Input: dimensioned drawing with shaded views. Units: mm. Origin: part minimum x, y, z. Give positions to 0.01 mm unless a question says otherwise; leave off trailing zeros. Loops run counter-clockwise (first coordinate to the right, second up) from the corner with the lowest first, then second, coordinate; pieces in that order, holes last.
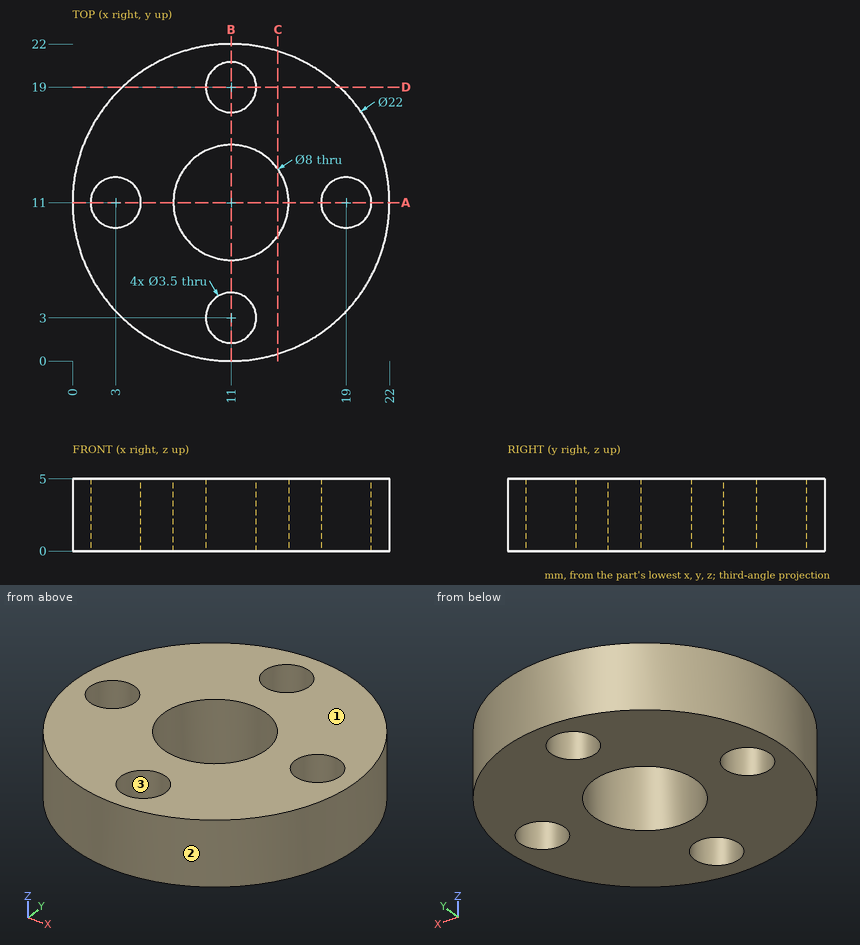
Item 1: Pin query (flat end, axial travel): pin 1 (2 mm diameter, centred on x = 6.5, z = 4, fed in from -Y); pin 2 (3 mm diameter, centred on x = 5.5, z = 1.5, fed in from -Y). Return the tip coordinate at first contact, or that it passes through.
Values follow:
pin 1: stops at y = 0.57
pin 2: stops at y = 0.75
Item 2: Ray query, probe 1 along Y at (x, z) = (11, 2.3); probe 2 along Y at (x, z) = (11.75, 4.05). Return the intervals inside material, ascending.
Values follow:
probe 1: y = 0 to 1.25, 4.75 to 7, 15 to 17.25, 20.75 to 22
probe 2: y = 0.03 to 1.42, 4.58 to 7.07, 14.93 to 17.42, 20.58 to 21.97
Item 3: Section query D-D on y = 19. Return loops of the section in (x, z).
Values follow:
outline: (3.45, 0) - (9.25, 0) - (9.25, 5) - (3.45, 5) - close; (12.75, 0) - (18.55, 0) - (18.55, 5) - (12.75, 5) - close
Item 4: Section query A-A on y = 11. Return loops of the section in (x, z).
Values follow:
outline: (0, 0) - (1.25, 0) - (1.25, 5) - (0, 5) - close; (4.75, 0) - (7, 0) - (7, 5) - (4.75, 5) - close; (15, 0) - (17.25, 0) - (17.25, 5) - (15, 5) - close; (20.75, 0) - (22, 0) - (22, 5) - (20.75, 5) - close
Item 5: Section query C-C on x = 14.25. Return loops of the section in (y, z), plus the area to 3 significant figures.
Values follow:
outline: (0.49, 0) - (8.67, 0) - (8.67, 5) - (0.49, 5) - close; (13.33, 0) - (21.51, 0) - (21.51, 5) - (13.33, 5) - close
area: 81.8 mm2
Item 6: Draft query along X for the marked faces 1, 2 and 3. Return one class per face: +X half, -X half, draft (parallel to the pull), parting line (faces both ways), or undercut.
Values follow:
face 1: draft
face 2: parting line
face 3: undercut
